from build123d import *

# Parameters (mm, degrees)
F1_DEPTH  = 26
F2_W      = 17
F2_H      = 6
F3_DEPTH  = 40.2
F4_R      = 3.5
F5_DEPTH  = 40.2
F6_R      = 1.5
F7_DEPTH  = 20.6
F8_R      = 2.9
F9_DEPTH  = 10.6
F10_R     = 1.5
F11_DEPTH = 40.2
F12_W     = 6
F12_H     = 12
F13_DEPTH = 6
F14_W     = 1
F14_H     = 8
F15_DEPTH = 1
F16_R     = 5


with BuildPart() as f1:
    # F0 (on Front) → F1 (new body)
    with BuildSketch(Plane.XZ):
        Polygon((0, 37), (0, 0), (40.2, 0), (40.2, 37), (30.2, 37), (30.2, 4.4), (10, 4.4), (10, 37), align=None)
    extrude(amount=F1_DEPTH)

    # F2 (on face) → F3 (cut, through all)
    with BuildSketch(Plane.YZ.offset(40.2)):
        with Locations((-13, 17.6)):
            Rectangle(F2_W, F2_H)
    extrude(amount=-F3_DEPTH, mode=Mode.SUBTRACT)

    # F4 (on face) → F5 (cut, through all)
    with BuildSketch(Plane.YZ.offset(40.2)):
        with Locations((-13, 29)):
            Circle(F4_R)
    extrude(amount=-F5_DEPTH, mode=Mode.SUBTRACT)

    # F6 (on face) → F7 (cut, through all)
    with BuildSketch(Plane(origin=(0, 0, 0), x_dir=(1, 0, 0), z_dir=(0, 0, -1))):
        with Locations((5, 13)):
            Circle(F6_R)
        with Locations((35.2, 13)):
            Circle(F6_R)
    extrude(amount=-F7_DEPTH, mode=Mode.SUBTRACT)

    # F8 (on face) → F9 (cut)
    with BuildSketch(Plane(origin=(0, 0, 0), x_dir=(1, 0, 0), z_dir=(0, 0, -1))):
        with Locations((5, 13)):
            Circle(F8_R)
        with Locations((35.2, 13)):
            Circle(F8_R)
    extrude(amount=-F9_DEPTH, mode=Mode.SUBTRACT)

    # F10 (on face) → F11 (cut, through all)
    with BuildSketch(Plane(origin=(0, 0, 0), x_dir=(0, -1, 0), z_dir=(-1, 0, 0))):
        with Locations((5, 29)):
            Circle(F10_R)
        with Locations((21, 29)):
            Circle(F10_R)
    extrude(amount=-F11_DEPTH, mode=Mode.SUBTRACT)

    # F12 (on face) → F13 (cut)
    with BuildSketch(Plane.XY.offset(37)):
        with Locations((5, -13)):
            Rectangle(F12_W, F12_H)
    extrude(amount=-F13_DEPTH, mode=Mode.SUBTRACT)

    # F14 (on face) → F15 (cut)
    with BuildSketch(Plane.XY.offset(31)):
        with Locations((5, -13)):
            Rectangle(F14_W, F14_H)
    extrude(amount=-F15_DEPTH, mode=Mode.SUBTRACT)

    # F16
    f16_edges = [f1.edges().sort_by_distance(p)[0] for p in [
        (5, -26, 37),
        (5, 0, 37),
        (35.2, 0, 37),
        (35.2, -26, 37),
    ]]
    fillet(f16_edges, radius=F16_R)


solid = f1.part
CAD build for the part. Positions are in the model's coordinates, mm. A direction names the side the tool comes from. Round coordinates to 2 decimals unless told otherwise and drop trailing zeros. Write each loop counter-clockwise with the first axis right and the second up, starting at its lowest first coordinate (ties: lowest second). Pieces come first, ordered by that corner, then holes.
(1) 3-axis set-ups, long thin cutter, end or side, ignore diameter. For faces 1 (the face through (34, -12.1, 12.6)), 2 (the face through (30.2, -13, 21)), 3 (the face through (35.13, -4.805, 30.487)), 4 (the face through (5.5, -16.6, 30.5)): which of +Z, -Z, +X, -X, +Y, -Y reach the whole face in a straight line?
(2) Mould opens along Z. For faces 5 (the face through (5, -2, 36)), 6 (the face through (36.4, -11.8, 10.6)), 7 (the face through (35, -15, 14.6)), 8 (the face through (5, -19, 34)) say: pulls with the +Z half, pulls with the -Z half, needs draft (parallel to the pull), parting line crosses it, or undercut.
(3) Slice it at D-D, the plane x = 35.2. Write the cut outline in (y, z), and give its area (3 significant figures).
(4) Slice it at B-B, the plane z = 29. Count the separate pieces of the cut face and the enclosed holes in it, and give its area (3 significant figures).
(5) Slice it at A-A, the plane z = 8. Write the cut outline in (x, y).
(6) Probe line 1 along Z through (x, y) = (37, -13); line 2 along X through (y, z) = (-17.75, 31.5); line 3 along Z through (x, y) = (38.25, -13). List the from-to ranges inside material, lowest first.
(7) Drop flat-ended pins along their axis: P1, Ø5, axis at x = 15.5, y = -22.5, coming from the +Z side; P2, Ø2.5, axis at x = 6, y = -17, coming from the +Z side. Give the stop position or say it passes through.
From the geometry:
1. face 1: -Z
1. face 2: +Z, +Y, -Y
1. face 3: +X, -X
1. face 4: +Z
2. face 5: pulls with the +Z half
2. face 6: pulls with the -Z half
2. face 7: undercut
2. face 8: needs draft
3. outline: (-26, 0) - (-15.9, 0) - (-15.9, 10.6) - (-14.5, 10.6) - (-14.5, 14.6) - (-21.5, 14.6) - (-21.5, 20.6) - (-4.5, 20.6) - (-4.5, 14.6) - (-11.5, 14.6) - (-11.5, 10.6) - (-10.1, 10.6) - (-10.1, 0) - (0, 0) - (0, 32) arc R5 ccw to (-5, 37) - (-21, 37) arc R5 ccw to (-26, 32) - close; hole circle Ø3 at (-21, 29); hole circle Ø7 at (-13, 29); hole circle Ø3 at (-5, 29)
3. area: 723 mm2
4. separate pieces: 8
4. enclosed holes: 0
4. area: 260 mm2
5. outline: (0, -26) - (10, -26) - (10, 0) - (0, 0) - close; (30.2, -26) - (40.2, -26) - (40.2, 0) - (30.2, 0) - close; hole circle Ø5.8 at (5, -13); hole circle Ø5.8 at (35.2, -13)
6. line 1: z = 10.6 to 14.6, 20.6 to 25.5, 32.5 to 37
6. line 2: x = 0 to 2, 8 to 10, 30.2 to 40.2
6. line 3: z = 0 to 14.6, 20.6 to 25.5, 32.5 to 37
7. P1: stops at z = 4.4
7. P2: stops at z = 31
